The drawing under review shows one solid part. Ordinate dimensions are in mm from its lowest x, y, z. A direction names the side the tool comes from. Give positions to 0.01 mm unless a question says otherwise; leave off trailing zeros. Write each loop counter-clockwise with the first axis right and the second up, starting at its lowest first coordinate (ties: lowest second). Pieces come first, ordered by that corner, then holes. Notation, with made-up numbers: (43.25, -19.75) -> (89.25, -19.75) arc R15 ccw to (89.25, -0.75) -> close; hole circle Ø4 at (81.5, 41). An arc over 180 degrees is marked (long way). Write item = value, one per line.
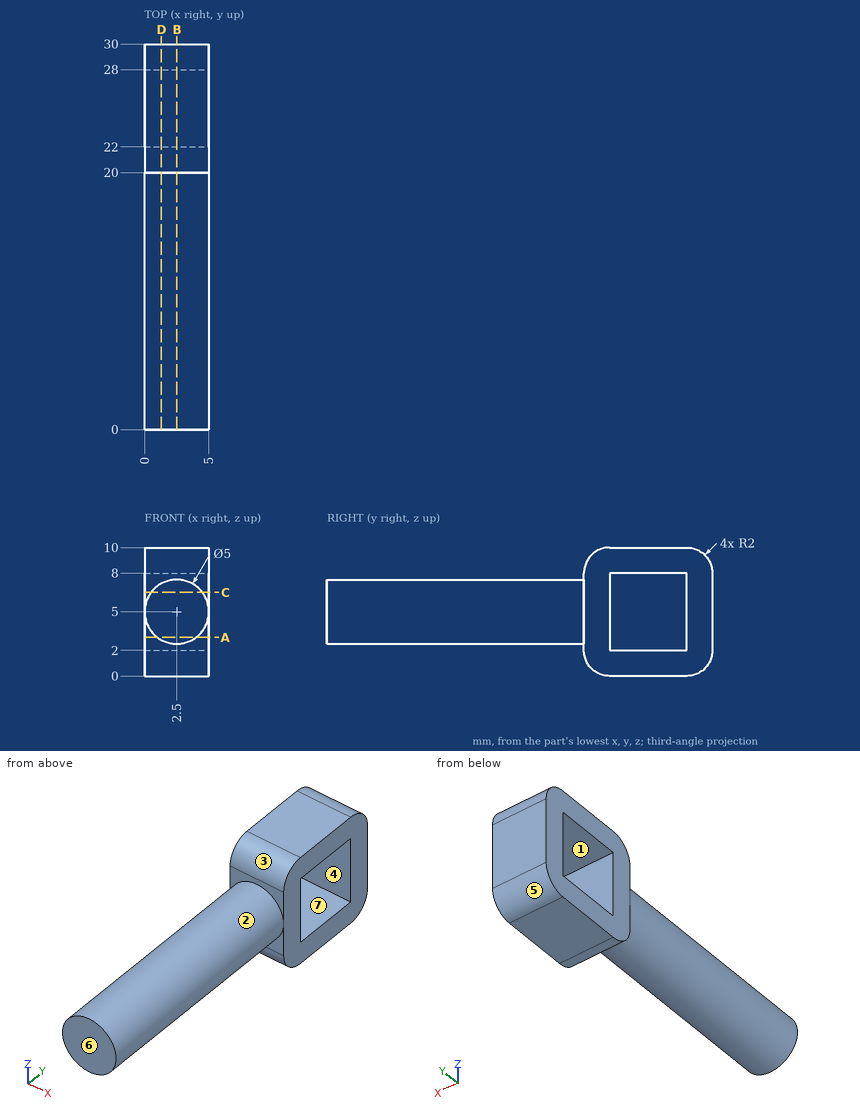
(1) Take a section at D-D (x = 1.3). Write out the cut boundary in (y, z).
Answers below:
outline = (0, 2.81) -> (20, 2.81) -> (20, 2) arc R2 ccw to (22, 0) -> (28, 0) arc R2 ccw to (30, 2) -> (30, 8) arc R2 ccw to (28, 10) -> (22, 10) arc R2 ccw to (20, 8) -> (20, 7.19) -> (0, 7.19) -> close; hole (22, 2) -> (28, 2) -> (28, 8) -> (22, 8) -> close
(2) The part is to be moulded in two halves that separate along Z. For the marked faces 4, 5, 6 and 7, say which applies: released by +Z, released by -Z, zero draft, split by the parting line, or undercut.
Answers below:
face_4 = undercut
face_5 = released by -Z
face_6 = zero draft
face_7 = undercut
(3) Tool access review of the marked faces 1, 2 and 3: name each direction out of +Z, -Z, +X, -X, +Y, -Y from which nothing blocks a thin tool from reaching the whole face with its end or side.
Answers below:
face_1 = +X, -X
face_2 = -Y
face_3 = +Z, +X, -X, -Y
(4) Take a section at A-A (z = 3). Write out the cut boundary in (x, y).
Answers below:
outline = (0, 20) -> (1, 20) -> (1, 0) -> (4, 0) -> (4, 20) -> (5, 20) -> (5, 22) -> (0, 22) -> close; (0, 28) -> (5, 28) -> (5, 30) -> (0, 30) -> close
(5) To check wall thickness, follow probe 1 along Y at (x, z) = (4.15, 4.5); probe 2 along Z at (x, y) = (3.85, 25); probe 3 along Z at (x, y) = (0.55, 14.75). State the ranges of each line that lie inside material, in increasing order.
Answers below:
probe_1 = 0 to 22, 28 to 30
probe_2 = 0 to 2, 8 to 10
probe_3 = 3.44 to 6.56
(6) Take a section at B-B (x = 2.5). Write out the cut boundary in (y, z).
Answers below:
outline = (0, 2.5) -> (20, 2.5) -> (20, 2) arc R2 ccw to (22, 0) -> (28, 0) arc R2 ccw to (30, 2) -> (30, 8) arc R2 ccw to (28, 10) -> (22, 10) arc R2 ccw to (20, 8) -> (20, 7.5) -> (0, 7.5) -> close; hole (22, 2) -> (28, 2) -> (28, 8) -> (22, 8) -> close
(7) For pin 1 (4 mm diameter, centred on y = 14, z = 2.5, fed in from +X); pin 2 (1.5 mm diameter, centred on x = 2.5, z = 8.5, fed in from -Y), all flat-tipped, find the tip position at first contact; note any pin that passes through.
Answers below:
pin_1 = 4.95
pin_2 = 20
(8) Take a section at C-C (z = 6.5). Write out the cut boundary in (x, y), plus the area to 3 significant figures.
Answers below:
outline = (0, 20) -> (0.5, 20) -> (0.5, 0) -> (4.5, 0) -> (4.5, 20) -> (5, 20) -> (5, 22) -> (0, 22) -> close; (0, 28) -> (5, 28) -> (5, 30) -> (0, 30) -> close
area = 100 mm^2
